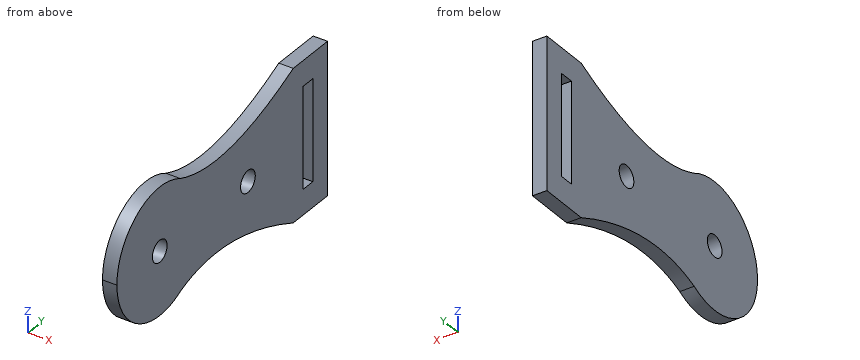
```python
from build123d import *

# Parameters (mm, degrees)
RESSALTO_EXTRUS_O1_DEPTH = 2
ESBO_O2_R                = 1.5
ESBO_O2_W                = 14
ESBO_O2_H                = 2
CORTE_EXTRUS_O1_DEPTH    = 3.0000001


with BuildPart() as part:
    # Esboço1 → Ressalto-extrusão1 (new body)
    with BuildSketch(Plane(origin=(0, 0, 0), x_dir=(0, 0, -1), z_dir=(1, 0, 0))):
        with BuildLine():
            Line((-10.5, 34.25), (0, 34.25))
            Line((0, 34.25), (0, -8.75))
            ThreePointArc((0, -8.75), (-7.522394047, -4.46946169), (-7.684811888, 4.184037075))
            add(Edge.make_bspline(
                [(-10.5, 27.25), (-3.865048066, 13.251366251), (-7.684811888, 4.184037075)],
                knots=[0, 0, 0, 0.912495845, 0.912495845, 0.912495845], degree=2))
            Line((-10.5, 27.25), (-10.5, 34.25))
        make_face()
    ressalto_extrus_o1 = extrude(amount=RESSALTO_EXTRUS_O1_DEPTH)

    # Espelhar1: Ressalto-extrusão1 across plane
    add(ressalto_extrus_o1.mirror(Plane(origin=(2, 34.25, 0), x_dir=(1, 0, 0), z_dir=(0, 0, 1))))

    # Esboço2 → Corte-extrusão1 (cut, through all)
    with BuildSketch(Plane(origin=(2, 0, 0), x_dir=(0, 0, -1), z_dir=(1, 0, 0))):
        with Locations((0, 18)):
            Circle(ESBO_O2_R)
        Circle(ESBO_O2_R)
        with Locations((0, 30.25)):
            Rectangle(ESBO_O2_W, ESBO_O2_H)
    extrude(amount=-CORTE_EXTRUS_O1_DEPTH, mode=Mode.SUBTRACT)


solid = part.part
```
Here's how the part is built. I have some questions about the finished solid (model axes, mm). Coordinates: 2 decimals unless noted, no trailing zeros. Write each loop counter-clockwise with the first axis right and the second up, starting at its lowest first coordinate (ties: lowest second). Pieces come first, ordered by that corner, then holes. Notation, with made-up numbers: M -21,5 L -12,5 A24 cw -12,30 Z; hole C 40.5,70 d7. An arc over 180 degrees is marked long. Answer as CSV lines item,"result". Start each with the question number.
Q1. Suppose I cut it at D-D, the plane x = 1.25. State how many separate pieces and enclosed holes the cut face has, then the cut area to 3 significant figures.
Q2. Suppose I cut it at A-A, the plane y = 0. List the corners of the cut face in (x, z) for me.
Q3. Will this pin go through, and if not, where does the flat tip stop? pin 1 Ø0.6 at (x, z) = (1, -1.5) entering from -Y.
Q4. I need wall thicknesses on probe 1 along Y at (x, z) = (0.4, 0); probe 2 along Y at (x, z) = (1.25, -1); probe 3 along Y at (x, z) = (0.9, 3.25). Which ranges of each line are inside material? Lowest first, please. Write a range as [from, to].
Q5. Suppose I cut it at B-B, the plane z = 0.5. List the corners of the cut face in (x, y) for me, then the cut area to 3 significant figures.
Q6. Suppose I cut it at C-C, the plane z = -5.5. List the corners of the cut face in (x, y) for me.
Entries:
1,separate pieces,"1"
1,enclosed holes,"3"
1,area,"639 mm²"
2,outline,"M 0,-8.75 L 2,-8.75 L 2,-1.5 L 0,-1.5 Z; M 0,1.5 L 2,1.5 L 2,8.75 L 0,8.75 Z"
3,pin 1,"stops at y = -8.67"
4,probe 1,"y = [-8.75, -1.5], [1.5, 16.5], [19.5, 29.25], [31.25, 34.25]"
4,probe 2,"y = [-8.69, -1.12], [1.12, 16.88], [19.12, 29.25], [31.25, 34.25]"
4,probe 3,"y = [-8.12, 29.25], [31.25, 34.25]"
5,outline,"M 0,-8.74 L 2,-8.74 L 2,-1.41 L 0,-1.41 Z; M 0,1.41 L 2,1.41 L 2,16.59 L 0,16.59 Z; M 0,19.41 L 2,19.41 L 2,29.25 L 0,29.25 Z; M 0,31.25 L 2,31.25 L 2,34.25 L 0,34.25 Z"
5,area,"70.7 mm²"
6,outline,"M 0,-6.81 L 2,-6.81 L 2,29.25 L 0,29.25 Z; M 0,31.25 L 2,31.25 L 2,34.25 L 0,34.25 Z"
